from build123d import *

# Parameters (mm, degrees)
F0_R     = 15
F0_R_2   = 7.5
F1_DEPTH = 4
F0_R_3   = 6
F2_DEPTH = 7.7
F3_SIZE  = 0.25


with BuildPart() as f1:
    # F0 (on Right) → F1 (new body)
    with BuildSketch(Plane.YZ):
        Circle(F0_R)
        Circle(F0_R_2, mode=Mode.SUBTRACT)
    extrude(amount=F1_DEPTH)

    # F0 (on Right) → F2 (join)
    with BuildSketch(Plane.YZ):
        Circle(F0_R_2)
        Circle(F0_R_3, mode=Mode.SUBTRACT)
    extrude(amount=F2_DEPTH)

    # F3
    f3_edges = [f1.edges().sort_by_distance(p)[0] for p in [
        (0, -15, 0),
        (0, -6, 0),
        (4, -15, 0),
        (7.7, -7.5, 0),
        (7.7, -6, 0),
    ]]
    chamfer(f3_edges, length=F3_SIZE)

    # F4 (on Front) → F5 (revolve, cut)
    with BuildSketch(Plane.XZ):
        with BuildLine():
            Line((4.5, 7.5), (4, 7.5))
            ThreePointArc((4, 7.5), (4.25, 7.291997), (4.5, 7.5))
        make_face()
    revolve(axis=Axis((2, 0, 0), (1, 0, 0)), mode=Mode.SUBTRACT)


solid = f1.part
Work out the finished part from the listing and answer in its coordinate system (mm). A direction names the side the tool comes from. Give positions to 0.01 mm unless a question says otherwise; leave off trailing zeros. Loops run counter-clockwise (first coordinate to the right, second up) from the corner with the lowest first, then second, coordinate; pieces in that order, holes last. Notation, with made-up numbers: (4, 49) - (14, 49) arc R18 cw to (14, 67) - close; hole circle Ø4 at (-7.5, 79.25). An arc over 180 degrees is marked (long way). Answer in a Markdown table with one row per item. Add a question column.
Q1. The part is cut by section A-A (z = 0). Determine the outline of the cut face in (x, y), and give its area (3 significant figures).
Q2. Determine the mould class of faces 1 (the cylindrical face through (4, -6, 0)), 2 (the flat face through (0, 6, -3)), 3 (the cylindrical face through (1.976, -14.985, 0.66)) for opening direction Y: released by +Y, released by -Y, zero draft, split by the parting line, or undercut.
Q3. Consider line 1 along Z through (x, y) = (3, 0); line 2 along Z through (x, y) = (5.75, 0); line 3 along X through (y, z) = (5, -6). Determine where each line is inside the solid, lowest interval first.
Q4. A tool of negligible diameter and unlimited length cuts with its end or side. For faces 4 (the flat face through (7.7, 0, 6.5)), 5 (the cylindrical face through (5.954, 7.154, 2.253)), from which of +Z, -Z, +X, -X, +Y, -Y can it reach the whole face along a straight path? Write none if from no direction.
Q5. Each of these flat-tipped pins is pushed along its axis until it touches: P1, Ø4, axis at x = 5, z = 7, coming from the -Y side; P2, Ø1, axis at x = 6.5, z = -2, coming from the -Y side; P3, Ø2, axis at x = 6, y = -3, coming from the -Z side. Where does it stop, or does it pass through?
Solution:
| question | item | result |
|---|---|---|
| 1 | outline | (0, -14.75) - (0.25, -15) - (3.75, -15) - (4, -14.75) - (4, -7.5) arc R0.25 cw to (4.5, -7.5) - (7.45, -7.5) - (7.7, -7.25) - (7.7, -6.25) - (7.45, -6) - (0.25, -6) - (0, -6.25) - close; (0, 6.25) - (0.25, 6) - (7.45, 6) - (7.7, 6.25) - (7.7, 7.25) - (7.45, 7.5) - (4.5, 7.5) arc R0.25 cw to (4, 7.5) - (4, 14.75) - (3.75, 15) - (0.25, 15) - (0, 14.75) - close |
| 1 | area | 82.6 mm² |
| 2 | face 1 | undercut |
| 2 | face 2 | zero draft |
| 2 | face 3 | split by the parting line |
| 3 | line 1 | z = -15 to -6, 6 to 15 |
| 3 | line 2 | z = -7.5 to -6, 6 to 7.5 |
| 3 | line 3 | x = 0 to 4 |
| 4 | face 4 | +Z, -Z, +X, +Y, -Y |
| 4 | face 5 | +X |
| 5 | P1 | stops at y = -13.98 |
| 5 | P2 | stops at y = -7.35 |
| 5 | P3 | stops at z = -7.23 |
